Autodesk Inventor part; units mm, degrees
ref_plane "YZ Plane" through (0, 0, 0) normal (1, 0, 0) x (0, 1, 0)
ref_plane "XZ Plane" through (0, 0, 0) normal (0, 1, 0) x (-1, 0, 0)
ref_plane "XY Plane" through (0, 0, 0) normal (0, 0, 1) x (1, 0, 0)
sketch "Sketch1" plane through (0, 0, 0) normal (0, 0, 1) x (1, 0, 0)
  line L0 (0, 0) -> (181.174, 0)
  line L1 (181.174, 0) -> (181.174, 350.17)
  line L2 (181.174, 350.17) -> (0, 350.17)
  line L3 (0, 350.17) -> (0, 0)
  dimension "d0" = 181.174
  dimension "d1" = 350.17
extrude "Plate1" add sketch "Sketch1" along normal blind 0.5
sketch "Sketch3" plane through (181.174, 0.5, 0) normal (0, -1, 0) x (1, 0, 0)
  line L0 (-181.174, 0) -> (0, 0)
  line L1 (0, 0) -> (0, 10)
  line L2 (0, 10) -> (-181.174, 10)
  line L3 (-181.174, 10) -> (-181.174, 0)
edge flange "Flange1" height 10 angle 90 thickness 0.5 bend radius 0.5 thickness toward (0, -1, 0) relief tear relief width 0.5 relief depth 0.25 edges at (90.587, 0, 0.5) wall of the first edge with corners at (0, 0.5, 0) (181.174, 0.5, 0) (181.174, 0.5, 10) (0, 0.5, 10)
bend "Bend1"
corner "Corner1"
sketch "Sketch4" plane through (0, 0, 0.5) normal (0, 0, 1) x (1, 0, 0)
  line L0 (181.174, 350.17) -> (181.174, 1)
  line L1 (10.4326, 171.5141) -> (10.4326, 6.5941)
  arc A0 (10.4326, 6.5941) -> (12.9726, 4.0541) centre (12.9726, 6.5941) ccw
  line L2 (177.8926, 4.0541) -> (12.9726, 4.0541)
  arc A1 (177.8926, 4.0541) -> (180.4326, 6.5941) centre (177.8926, 6.5941) ccw
  line L3 (180.4326, 171.5141) -> (180.4326, 6.5941)
  arc A2 (180.4326, 171.5141) -> (177.8926, 174.0541) centre (177.8926, 171.5141) ccw
  line L4 (177.8926, 174.0541) -> (12.9726, 174.0541)
  arc A3 (12.9726, 174.0541) -> (10.4326, 171.5141) centre (12.9726, 171.5141) ccw
  circle A4 centre (174.0826, 14.2141) radius 2.032
  circle A5 centre (174.0826, 169.1541) radius 2.032
  circle A6 centre (16.6026, 169.1541) radius 2.032
  circle A7 centre (16.6026, 37.0741) radius 2.032
  line L5 (181.174, 0) -> (181.174, 10.5)
  line L6 (181.174, 1) -> (181.174, 350.17)
  line L7 (181.174, 10.5) -> (174.824, 10.5) construction
  circle A8 centre (174.824, 10.5) radius 1.5
  line L8 (174.824, 10.5) -> (17.344, 10.5) construction
  line L9 (17.344, 10.5) -> (17.344, 33.36) construction
  circle A9 centre (17.344, 33.36) radius 1.5
  line L10 (17.344, 33.36) -> (17.344, 165.44) construction
  circle A10 centre (17.344, 165.0277) radius 1.5
  line L11 (174.824, 10.5) -> (174.824, 165.44) construction
  circle A11 centre (174.824, 165.44) radius 1.5
  point P0 (0, 0)
  point P1 (95.4326, 89.0541)
  dimension "d26" = 10.5
  dimension "d27" = 6.35
  dimension "d28" = 3
  dimension "d29" = 157.48
  dimension "d30" = 22.86
  dimension "d31" = 3
  dimension "d32" = 132.08
  dimension "d33" = 3
  dimension "d34" = 154.94
  dimension "d35" = 3
extrude "Extrusion2" cut sketch "Sketch4" against normal blind 10 contours A8 | A9 | A10 | A11
sketch "Sketch5" plane through (0, 0, 0.5) normal (0, 0, 1) x (1, 0, 0)
  circle A0 centre (17.344, 165.0277) radius 1.5
  line L0 (0, 1) -> (0, 350.17)
  line L1 (17.344, 165.0277) -> (17.344, 131.5227) construction
  line L2 (17.344, 131.5227) -> (17.344, 43.5207) construction
  line L3 (17.344, 131.5227) -> (10.994, 131.5227) construction
  line L4 (10.994, 131.5227) -> (0, 131.5227)
  line L5 (0, 131.5227) -> (0, 43.5207)
  line L6 (0, 43.5207) -> (10.994, 43.5207)
  line L7 (10.994, 43.5207) -> (10.994, 131.5227)
  line L8 (10.994, 131.5227) -> (0, 131.5227)
  line L9 (0, 131.5227) -> (0, 141.5227)
  line L10 (0, 141.5227) -> (10.994, 141.5227)
  line L11 (10.994, 141.5227) -> (10.994, 131.5227)
  line L12 (0, 43.5207) -> (10.994, 43.5207)
  line L13 (10.994, 43.5207) -> (10.994, 38.5207)
  line L14 (10.994, 38.5207) -> (0, 38.5207)
  line L15 (0, 38.5207) -> (0, 43.5207)
  point P0 (0, 0)
  dimension "d38" = 33.505
  dimension "d39" = 88.002
  dimension "d40" = 6.35
  dimension "d43" = 10
  dimension "d44" = 5
extrude "Extrusion4" cut sketch "Sketch5" against normal blind 10 contours L0 L6 L13 L14 | L0 L4 L7 L6 | L0 L10 L11 L4
equation "\"d2\" = Thickness"
equation "\"d16\" = BendReliefWidth"
equation "\"d17\" = BendReliefDepth"
equation "\"d18\" = MinimumRemnant"
equation "\"d19\" = TransitionRadius"
equation "\"d22\" = BendRadius"
equation "\"d23\" = CornerReliefSize"
equation "\"d24\" = GapSize"
equation "\"d25\" = JacobiRadiusSize"
equation "\"BendRadius\" = Thickness"
equation "\"BendReliefWidth\" = Thickness"
equation "\"BendReliefDepth\" = 0.5 * Thickness"
equation "\"CornerReliefSize\" = 4 * Thickness"
equation "\"MinimumRemnant\" = 2 * Thickness"
equation "\"TransitionRadius\" = BendRadius"
equation "\"JacobiRadiusSize\" = BendRadius"
equation "\"GapSize\" = Thickness"
properties part number "my trunk"
Geometry check sheet. Reference: the model listing, model coordinates, mm. A direction names the side the tool comes from. Coordinates: 2 decimals unless noted, no trailing zeros. Order: outer loops, then holes, each group sorted by start corner. A loop starts at its lowest first (then second) coordinate and runs counter-clockwise, first axis right, second up. Notation, with made-up numbers: (83.25, 82.5) -> (92.25, 82.5) arc R35 ccw to (92.25, 121.5) -> close; hole circle Ø4 at (9.25, 37). An arc over 180 degrees is marked (long way). Use a Markdown table: item, result. Add a question column.
1. Cross-section at B-B (y = 44.5). Enter the section's corners in (x, z).
2. Cross-section at A-A (x = 137). Enter the section's corners in (y, z), and give its area (3 significant figures).
3. Cross-section at C-C (z = 6.75). Enter the section's corners in (x, y), and give its area (3 significant figures).
4. Go/stop test with flat-tipped pins: pin 1 Ø4.5 at (x, z) = (100.5, 6) entering from +Y; pin 2 Ø1.5 at (x, y) = (114.5, 122) entering from +Z; pin 3 Ø2.5 at (x, y) = (174.824, 10.5) entering from +Z; pin 4 Ø6 at (x, z) = (75.5, 1.5) entering from -Y. Record where each tip stops, or that it passes through.
5. Set-up check for faces 1 (the face through (89, 178, 0.5)), 2 (the face through (181.174, 174.3, 0.2)): record each of +Z, -Z, +X, -X, +Y, -Y from which the full face is reachable in a straight line by a thin tool's end or side.
6. Material ranges on L1, parallel to X at y = 165.44, z = 0.4; L2, parallel to Z at x = 39.5, y = 215, recorded low to high.
Filled sheet:
| question | item | result |
|---|---|---|
| 1 | outline | (10.99, 0) -> (181.17, 0) -> (181.17, 0.5) -> (10.99, 0.5) -> close |
| 2 | outline | (0, 1) arc R1 ccw to (1, 0) -> (350.17, 0) -> (350.17, 0.5) -> (1, 0.5) arc R0.5 cw to (0.5, 1) -> (0.5, 10) -> (0, 10) -> close |
| 2 | area | 180 mm2 |
| 3 | outline | (0, 0) -> (181.17, 0) -> (181.17, 0.5) -> (0, 0.5) -> close |
| 3 | area | 90.6 mm2 |
| 4 | pin 1 | y = 0.5 |
| 4 | pin 2 | z = 0.5 |
| 4 | pin 3 | through |
| 4 | pin 4 | y = 0 |
| 5 | face 1 | +Z, +X, -X, +Y |
| 5 | face 2 | +Z, -Z, +X, +Y, -Y |
| 6 | L1 | 0 to 15.9, 18.79 to 173.32, 176.32 to 181.17 |
| 6 | L2 | 0 to 0.5 |
